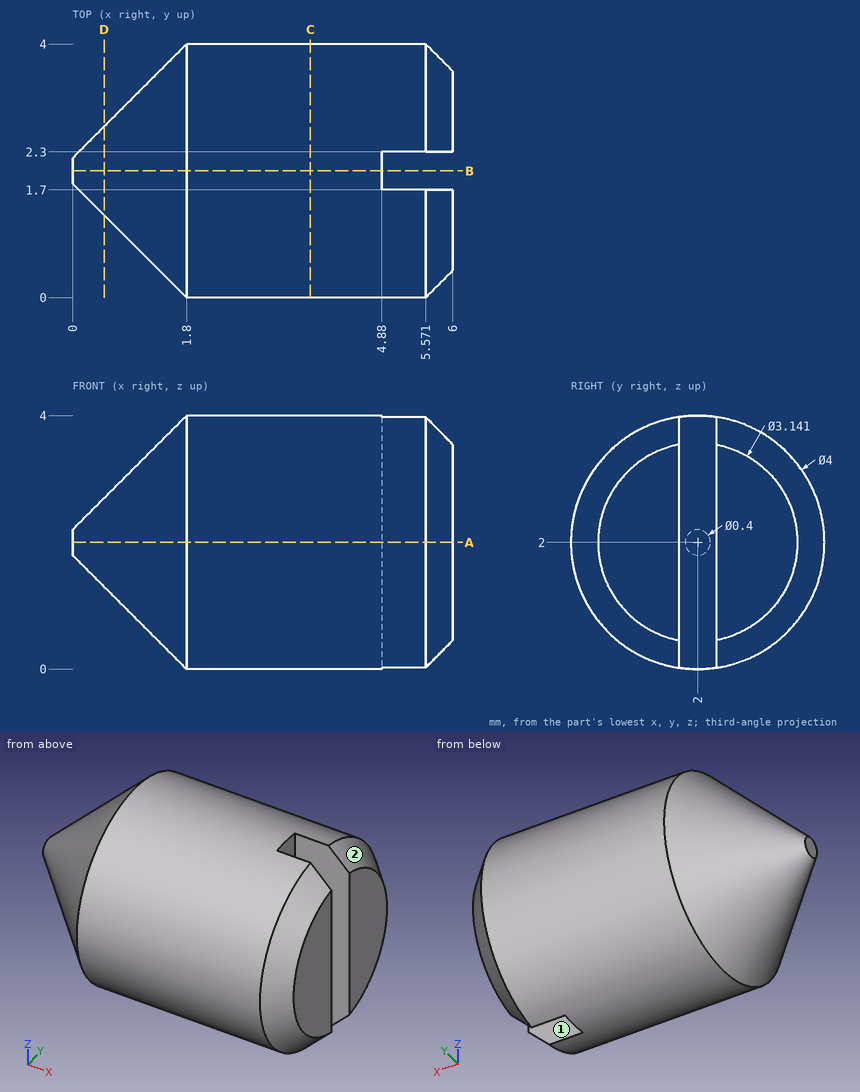
Could you check a few things on this drawing? It's one solid part, dimensions in mm from its lowest x, y, z. A direction names the side the tool comes from. Give positions to 0.01 mm unless a question says otherwise; leave off trailing zeros. Write each loop counter-clockwise with the first axis right and the second up, starting at its lowest first coordinate (ties: lowest second). Pieces come first, ordered by that corner, then holes.
(1) Imagine slicing it at C-C, the plane x = 3.75. Write out the boundary of the cut face in (y, z).
Output values:
outline: circle Ø4 at (2, 2)
(2) Will these pins go through, and if not, where does the flat tip stop? pin 1 (1 mm diameter, centred on x = 1, y = 2, fed in from -Z); pin 2 (2 mm diameter, centred on x = 5, z = 0.5, fed in from +Y); pin 3 (0.9 mm diameter, centred on x = 5, z = 1.5, fed in from -Y).
Output values:
pin 1: stops at z = 0.3
pin 2: stops at y = 3.94
pin 3: stops at y = 0
(3) If I drill on L1, parallel to Z at x = 4.25, y = 1.7; L2, parallel to Y at x = 5.75, z = 0.85, over which ranges is the centre line in solid material (lowest first)?
Output values:
L1: z = 0.02 to 3.98
L2: y = 0.59 to 1.7, 2.3 to 3.41
(4) Imagine slicing it at B-B, the plane y = 2. Write out the boundary of the cut face in (x, z).
Output values:
outline: (0, 1.8) - (1.8, 0) - (4.88, 0) - (4.88, 4) - (1.8, 4) - (0, 2.2) - close
(5) Imagine slicing it at A-A, the plane z = 2. Write out the boundary of the cut face in (x, y), and give its area (3 significant figures).
Output values:
outline: (0, 1.8) - (1.8, 0) - (5.57, 0) - (6, 0.43) - (6, 1.7) - (4.88, 1.7) - (4.88, 2.3) - (6, 2.3) - (6, 3.57) - (5.57, 4) - (1.8, 4) - (0, 2.2) - close
area: 19.9 mm2
(6) On a 3-axis mill with a long thin cutter (end or side, diameter ignored), from which of +Z, -Z, +X, -X, +Y, -Y can I reach the whole of each face in a straight line? I mean the marked faces 1 and 2. Say none if no direction works.
Output values:
face 1: +Z, -Z, +X
face 2: +X, +Y
(7) Imagine slicing it at D-D, the plane x = 0.5. Write out the boundary of the cut face in (y, z).
Output values:
outline: circle Ø1.4 at (2, 2)
